Answer from the drawing. Dimensions are ordinates in mm from the lowest x, y and z of the part. A direction names the side the tool comes from. Round coordinates to 2 decimals unless told otherwise and drop trailing zeros. Write each loop counter-clockwise with the first axis right and the second up, starting at its lowest first coordinate (ties: lowest second). Pieces come first, ordered by that corner, then holes. Notation, with made-up numbers: (36.25, 18) -> (83.25, 18) arc R10 ccw to (83.25, 28) -> close; hole circle Ø1 at (-15.5, -3.75). An arc over 180 degrees is marked (long way). Return JSON: item names as keys, results as strings. Group by question number.
(1) A cutting plane is placed at B-B on x = 15. Give the vertices of the cut face in (y, z), then the cut area to 3 significant figures.
(2) Straight lines are drawn through the part: line 1 (Y direction, x = 26.25, z = 3.5); line 2 (Y direction, x = 7, z = 4); line 3 (Y direction, x = 27.5, z = 26). For each, find the intervals that lie inside material, in ascending order.
(3) For the marked faces 1, 2 and 3, determine the directions among +Z, -Z, +X, -X, +Y, -Y from which every point of the face is accessible in a straight line to the end or side of a thin tool.
(4) A cutting plane is placed at D-D on y = 57. Give the vertices of the cut face in (x, z), then the cut area to 3 significant figures.
(5) Given pin 1 (12 mm diameter, centred on x = 17.5, z = 40.5, fed in from +Y); pin 2 (3 mm diameter, centred on y = 57, z = 4, fed in from -X); pin 3 (9 mm diameter, centred on x = 20, z = 35, fed in from +Y); pin 4 (9 mm diameter, centred on x = 12, y = 26.5, fed in from +Z), each flat-ended and moving along its own axis, determine where each tip first touches the part or whether it passes through.
(6) The mould has two halves that part along X. Classify the marked faces 4, 5 and 6: released by +X, released by -X, zero draft, split by the parting line, or undercut.
(7) A cutting plane is placed at C-C on y = 30.5. Give the vertices of the cut face in (x, z), then the cut area to 3 significant figures.
(8) A cutting plane is placed at A-A on z = 44. Give the vertices of the cut face in (x, y).
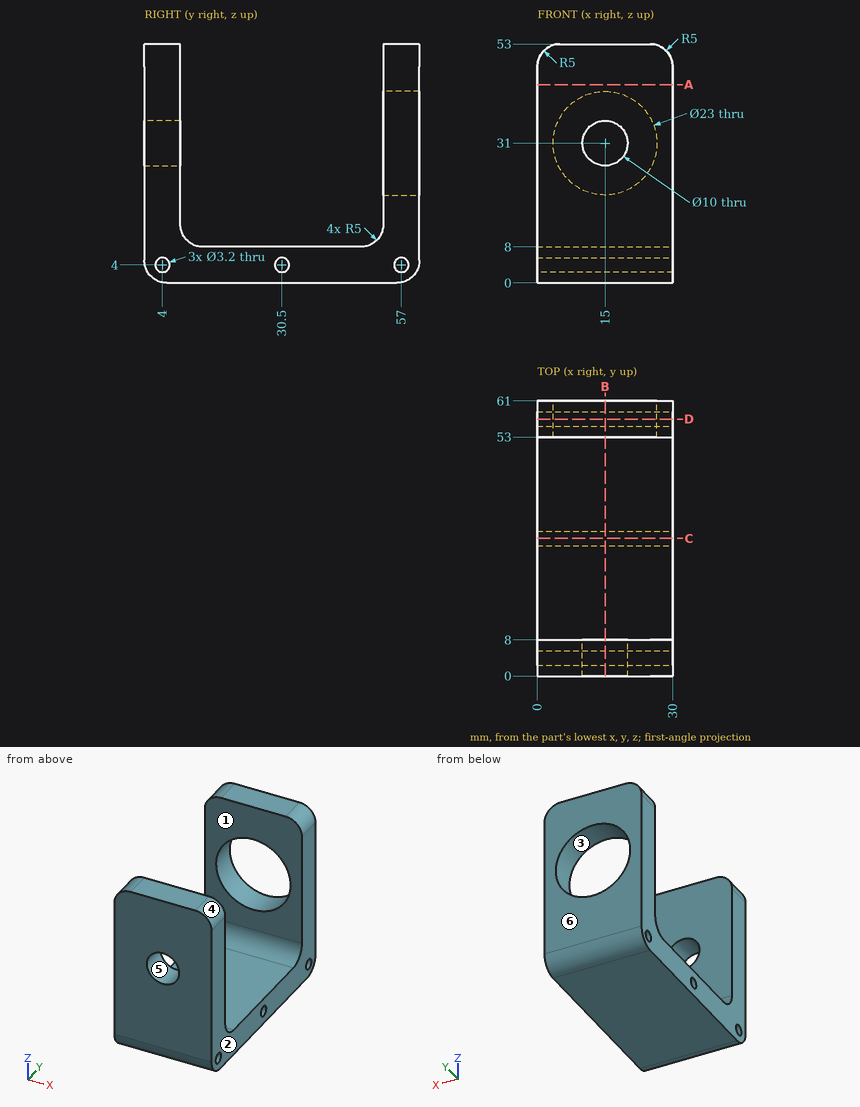
Checks:
{
 "1": {"outline": "(0, 5) arc R5 ccw to (5, 0) -> (56, 0) arc R5 ccw to (61, 5) -> (61, 19.5) -> (53, 19.5) -> (53, 13) arc R5 cw to (48, 8) -> (13, 8) arc R5 cw to (8, 13) -> (8, 26) -> (0, 26) -> close; (0, 36) -> (8, 36) -> (8, 53) -> (0, 53) -> close; (53, 42.5) -> (61, 42.5) -> (61, 53) -> (53, 53) -> close; hole circle Ø3.2 at (4, 4); hole circle Ø3.2 at (30.5, 4); hole circle Ø3.2 at (57, 4)", "area": "920 mm^2"},
 "2": {"line 1": "y = 0.23 to 2.48, 5.52 to 28.98, 32.02 to 55.48, 58.52 to 60.77", "line 2": "y = 0.1 to 2.4, 5.6 to 28.9, 32.1 to 55.4, 58.6 to 60.9", "line 3": "y = 0 to 8, 53 to 61"},
 "3": {"face 1": "+Z, +X, -X", "face 2": "+Z, -Z, +X, +Y, -Y", "face 3": "+Y"},
 "4": {"outline": "(0, 0.1) -> (30, 0.1) -> (30, 2.4) -> (0, 2.4) -> close; (0, 5.6) -> (30, 5.6) -> (30, 48) arc R5 ccw to (25, 53) -> (5, 53) arc R5 ccw to (0, 48) -> close; hole circle Ø23 at (15, 31)", "area": "1,060 mm^2"},
 "5": {"pin 1": "stops at y = 61", "pin 2": "passes through", "pin 3": "stops at y = 8", "pin 4": "stops at z = 8"},
 "6": {"face 4": "released by +X", "face 5": "undercut", "face 6": "zero draft"},
 "7": {"outline": "(0, 0) -> (30, 0) -> (30, 2.4) -> (0, 2.4) -> close; (0, 5.6) -> (30, 5.6) -> (30, 8) -> (0, 8) -> close", "area": "144 mm^2"},
 "8": {"outline": "(0, 0) -> (30, 0) -> (30, 8) -> (0, 8) -> close; (0, 53) -> (30, 53) -> (30, 61) -> (0, 61) -> close"}
}
